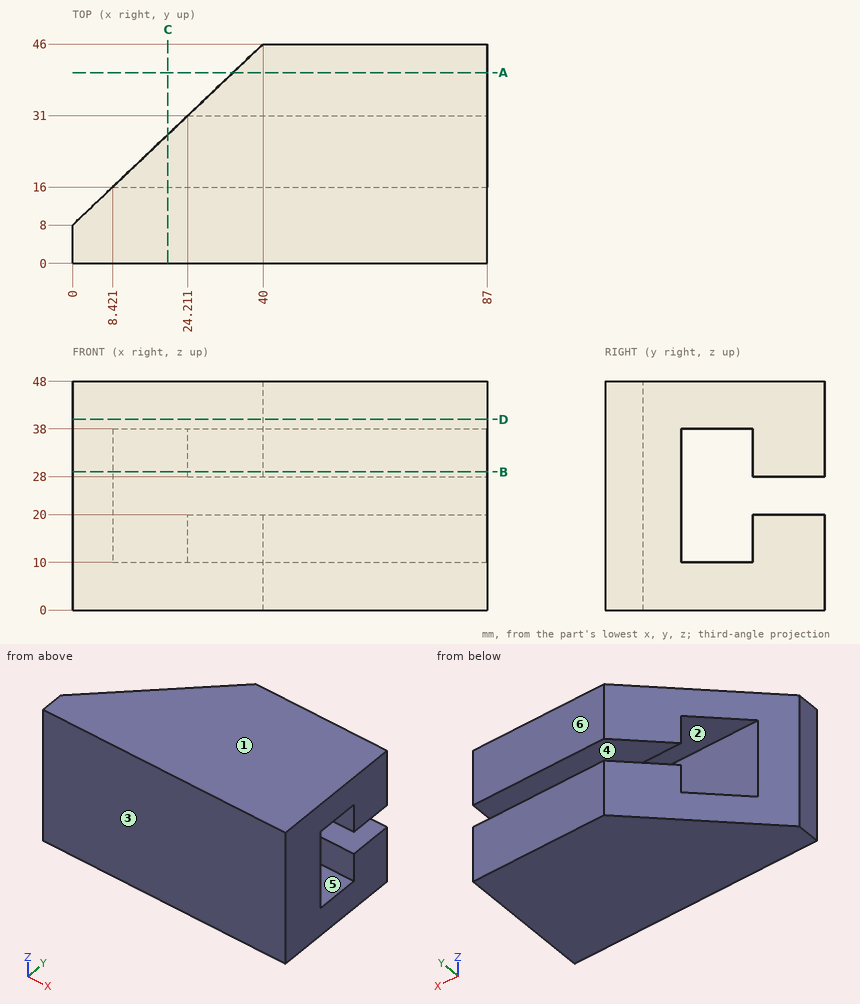
Print and shaded views of the part. All mm, measured from the part's lowest x, y and z. A direction names the side the tool comes from. Give positions to 0.01 mm unless a question says otherwise; leave off trailing zeros. Write each loop counter-clockwise with the first axis right and the second up, starting at its lowest first coordinate (ties: lowest second). Pieces come first, ordered by that corner, then holes. Notation, with made-up numbers: (68.25, 15.25) - (103.25, 15.25) arc R20 cw to (103.25, 26.25) - close; hole circle Ø7 at (-19, -5). An arc over 180 degrees is marked (long way). One line per question, with ' | ' between items. Start each with the question number.
(1) Pin check, flat tip, straight feed: P1, Ø3, axis at x = 23, z = 7, coming from the +Y side (1 decimal). Stop position of the tip, or through.
(2) Slice it at A-A on y = 40. Write the cut outline in (x, z) (1 decimal), plus the area to 3 significant figures.
(3) Wall check: line 1 along Z through (x, y) = (55.5, 30); line 2 along Z through (x, y) = (26, 32); line 3 along Y through (x, z) = (66.5, 17.5). Give the ranges that are in metal, low to high. Write a range as from..to.
(4) 3-axis set-ups, long thin cutter, end or side, ignore diameter. For the marked faces 4, 5 and 6: which of +Z, -Z, +X, -X, +Y, -Y reach the whole face in a straight line?
(5) Slice it at B-B on z = 29. Write the cut outline in (x, y), plus the area to 3 significant figures.
(6) Slice it at D-D on z = 40. Write the cut outline in (x, y).
(7) Two-plate mould, pull along Z, no slides. Class the marked faces 1, 2 and 3: +Z half, -Z half, draft (parallel to the pull), parting line (faces both ways), or undercut.
(8) Slice it at C-C on x = 20. Write the cut outline in (y, z).
Results below:
1) P1: y = 31.3
2) outline: (33.7, 0) - (87, 0) - (87, 20) - (33.7, 20) - close; (33.7, 28) - (87, 28) - (87, 48) - (33.7, 48) - close | area: 2,130 mm^2
3) line 1: 0..10, 38..48 | line 2: 0..20, 28..48 | line 3: 0..16, 31..46
4) face 4: +X, -X, +Y | face 5: +X, -X | face 6: +Z, -Z, +X, -X, +Y
5) outline: (0, 0) - (87, 0) - (87, 16) - (8.42, 16) - (0, 8) - close; (24.21, 31) - (87, 31) - (87, 46) - (40, 46) - close | area: 2,180 mm^2
6) outline: (0, 0) - (87, 0) - (87, 46) - (40, 46) - (0, 8) - close
7) face 1: +Z half | face 2: undercut | face 3: draft
8) outline: (0, 0) - (27, 0) - (27, 10) - (16, 10) - (16, 38) - (27, 38) - (27, 48) - (0, 48) - close
